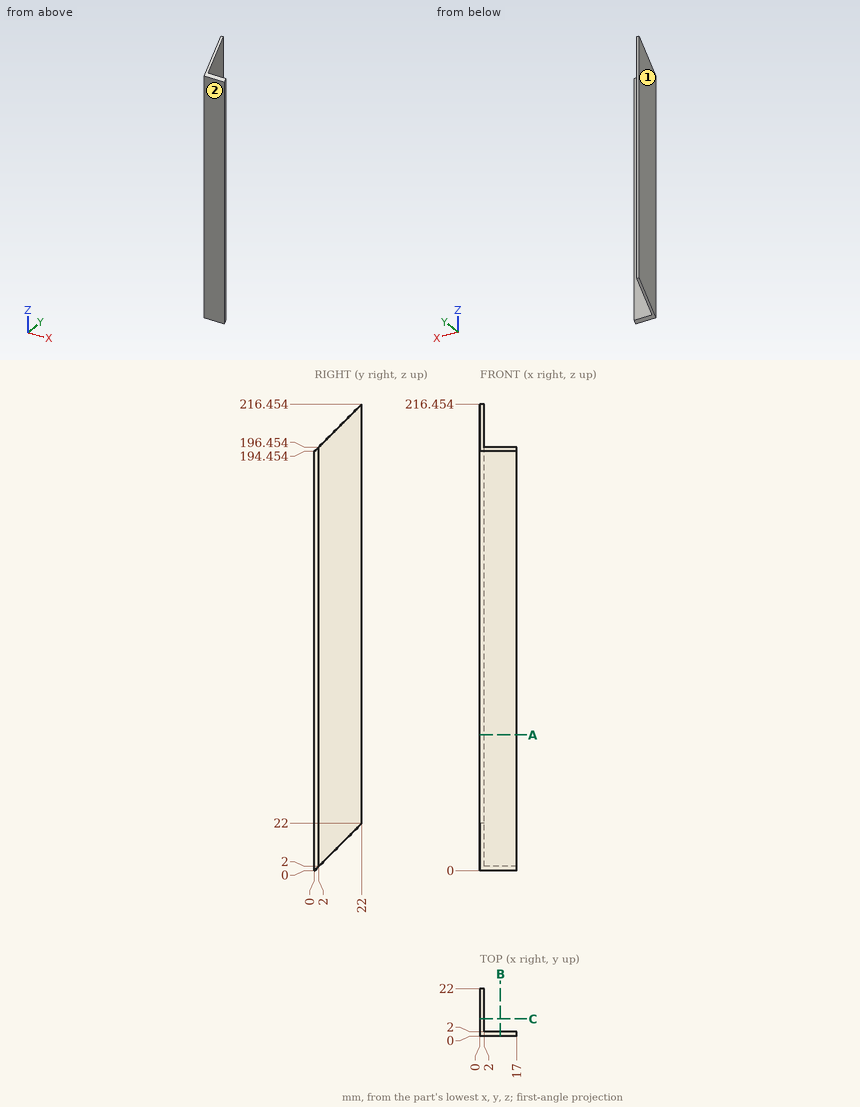
Verification items for this drawing (mm, ordinates from the low corner). Round coordinates to 2 decimals unless told otherwise and drop trailing zeros. Order: outer loops, then holes, each group sorted by start corner. A loop starts at its lowest first (then second) coordinate and runs counter-clockwise, first axis right, second up.
1) Cross-section at A-A, the plane z = 63. Record the cut outline in (x, y).
Geometry says:
outline: (0, 0) - (17, 0) - (17, 2) - (2, 2) - (2, 22) - (0, 22) - close
2) Depth check by flat-ended pin: pin 1 (4 mm diameter, centred on x = 11.5, z = 28.5, fed in from +Y). Enter the tip coordinate at first touch or a pass-through.
Geometry says:
pin 1: stops at y = 2
3) Draft check along X on the marked faces 1 and 2. Enter one of: +X half, -X half, draft (parallel to the pull), parting line (faces both ways), or undercut.
Geometry says:
face 1: -X half
face 2: draft
4) Cross-section at B-B, the plane x = 9.5. Record the cut outline in (y, z) (1 decimal).
Geometry says:
outline: (0, 0) - (2, 2) - (2, 196.5) - (0, 194.5) - close
5) Cross-section at C-C, the plane y = 8. Record the cut outline in (x, z) (1 decimal), plus the area to 3 significant figures.
Geometry says:
outline: (0, 8) - (2, 8) - (2, 202.5) - (0, 202.5) - close
area: 389 mm2
6) Material ranges on line 1 (Y direction, x = 6, z = 19.5); line 2 (Z direction, x = 1.25, y = 20) (1 decimal), recorded low to high.
Geometry says:
line 1: y = 0 to 2
line 2: z = 20 to 214.5
